The figure shows three views and two pictorial views of one solid part (mm, origin at its lowest corner). Answer the questions. A direction names the side the tool comes from. Round coordinates to 2 decimals unless told otherwise and drop trailing zeros. Loops run counter-clockwise (first coordinate to the right, second up) from the corner with the lowest first, then second, coordinate; pieces in that order, holes last. Notation, with made-up numbers: (33.5, -9.5) -> (44.5, -9.5) arc R27 cw to (44.5, 12.5) -> close; hole circle Ø7 at (4, 70). An arc over 180 degrees is marked (long way). Use a Markdown table: item, result. Add a question column.
Q1. Section D-D on z = 40 is taken. Give the vertices of the cut face in (x, y), then the cut area to 3 significant figures.
Q2. Section B-B on z = 52 is taken. Give the vertices of the cut face in (x, y), then the cut area to 3 significant figures.
Q3. Consider line 1 (Z direction, x = 28, y = 23.5); line 2 (X direction, y = 64.5, z = 70.5) (1 decimal); line 3 (X direction, y = 88.5, z = 16). Determine where each line is inside the solid, lowest interval first.
Q4. Which of the six approach directions +Z, -Z, +X, -X, +Y, -Y give full straight-line access (tool end or side, diameter ignored) to the marked faces 1, 2, 3, 4 and 5?
Q5. Given pin 1 Ø5 at (x, z) = (97, 32.5) entering from -Y; pin 2 Ø18.5 at (y, z) = (51, 72) entering from +X; pin 3 Ø4.5 at (y, z) = (28, 56.5) entering from +X; pin 4 Ø10 at (x, y) = (29.5, 73) entering from -Z, each flat-ended and moving along its own axis, determine where each tip first touches the part or whether it passes through.
Q6. Section A-A on y = 91 is taken. Give the vertices of the cut face in (x, z) (1 decimal), then the cut area to 3 significant figures.
Q7. Section C-C on x = 43 is taken. Give the vertices of the cut face in (y, z).
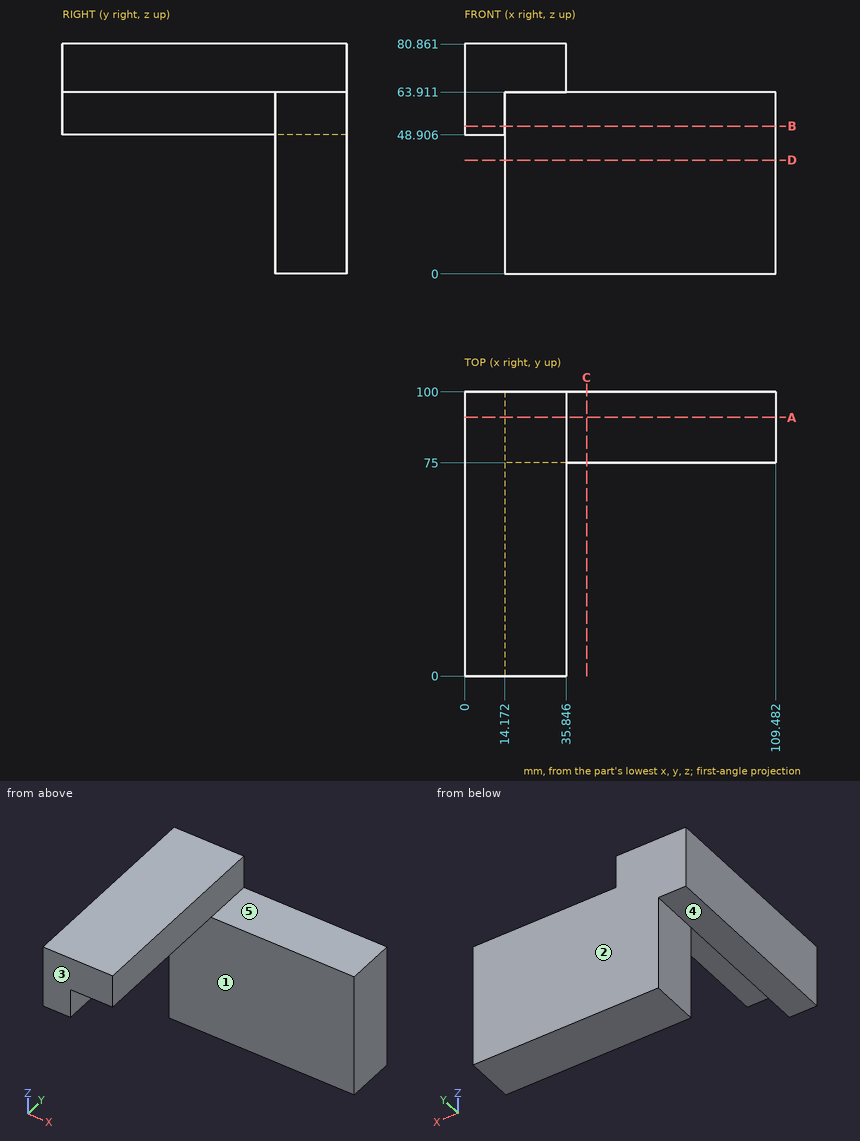
Checked values:
| question | item | result |
|---|---|---|
| 1 | outline | (14.17, 75) -> (109.48, 75) -> (109.48, 100) -> (14.17, 100) -> close |
| 1 | area | 2,380 mm2 |
| 2 | outline | (0, 0) -> (14.17, 0) -> (14.17, 75) -> (109.48, 75) -> (109.48, 100) -> (0, 100) -> close |
| 2 | area | 3,800 mm2 |
| 3 | line 1 | z = 63.91 to 80.86 |
| 3 | line 2 | x = 0 to 35.8 |
| 3 | line 3 | x = 14.17 to 109.48 |
| 4 | face 1 | -Z, +X, -Y |
| 4 | face 2 | +Z, -Z, +X, -X, +Y |
| 4 | face 3 | +Z, -Z, +X, -X, -Y |
| 4 | face 4 | -Z, -X, +Y, -Y |
| 4 | face 5 | +Z, +X, +Y, -Y |
| 5 | pin 1 | stops at y = 75 |
| 5 | pin 2 | stops at x = 35.85 |
| 5 | pin 3 | stops at x = 14.17 |
| 5 | pin 4 | stops at z = 0 |
| 6 | outline | (0, 48.9) -> (14.2, 48.9) -> (14.2, 0) -> (109.5, 0) -> (109.5, 63.9) -> (35.8, 63.9) -> (35.8, 80.9) -> (0, 80.9) -> close |
| 6 | area | 6,910 mm2 |
| 7 | outline | (75, 0) -> (100, 0) -> (100, 63.91) -> (75, 63.91) -> close |
